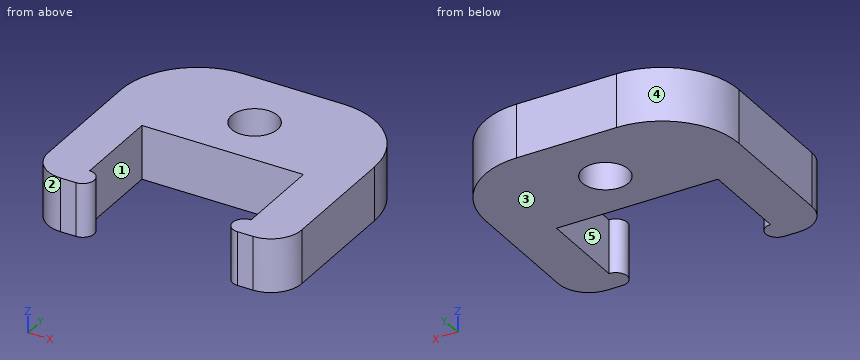
from build123d import *

# Parameters (mm, degrees)
SKETCH1_R           = 1.5
BOSS_EXTRUDE1_DEPTH = 3.5
FILLET1_R           = 2
FILLET2_R           = 5


with BuildPart() as part:
    # Sketch1 → Boss-Extrude1 (new body)
    with BuildSketch(Plane.XY):
        with BuildLine():
            Line((0, 15), (16.5, 15))
            Line((16.5, 15), (16.5, 0))
            Line((16.5, 0), (13.5, 0))
            ThreePointArc((13.5, 0), (12.75, 0.75), (13.5, 1.5))
            Line((13.5, 1.5), (13.5, 7.25))
            Line((13.5, 7.25), (3, 7.25))
            Line((3, 7.25), (3, 1.5))
            ThreePointArc((3, 1.5), (3.75, 0.75), (3, 0))
            Line((3, 0), (0, 0))
            Line((0, 0), (0, 15))
        make_face()
        with Locations((8.25, 10.75)):
            Circle(SKETCH1_R, mode=Mode.SUBTRACT)
    extrude(amount=BOSS_EXTRUDE1_DEPTH)

    # Fillet1
    fillet1_edges = [part.edges().sort_by_distance(p)[0] for p in [
        (16.5, 0, 1.75),
        (0, 0, 1.75),
    ]]
    fillet(fillet1_edges, radius=FILLET1_R)

    # Fillet2
    fillet2_edges = [part.edges().sort_by_distance(p)[0] for p in [
        (0, 15, 1.75),
        (16.5, 15, 1.75),
    ]]
    fillet(fillet2_edges, radius=FILLET2_R)


solid = part.part
Can you work these out from the model? Positions are in its coordinate system, mm. Face numbers are marked on the shaded views. A direction names the side the tool comes from. Give positions to 0.01 mm unless a question says otherwise; leave off trailing zeros. Loops run counter-clockwise (first coordinate to the right, second up) from the corner with the lowest first, then second, coordinate; pieces in that order, holes last. Notation, with made-up numbers: (17, 8.25) -> (50, 8.25) arc R16 cw to (50, 20.25) -> close; hole circle Ø1 at (32.5, 86.5). An arc over 180 degrees is marked (long way). Return JSON: item names as keys, results as strings.
Q1. For pin 1 Ø2.5 at (x, y) = (8.25, 10.75) entering from +Z, with a flat end and sliding along its axis, tell me the tip position at first contact or that it passes through.
Checks:
{"pin 1": "passes through"}
Q2. I want a section at A-A, the plane y = 4. List the corners of the cut face in (x, z) for me.
Checks:
{"outline": "(0, 0) -> (3, 0) -> (3, 3.5) -> (0, 3.5) -> close; (13.5, 0) -> (16.5, 0) -> (16.5, 3.5) -> (13.5, 3.5) -> close"}
Q3. I want a section at B-B, the plane z = 2.35. List the corners of the cut face in (x, y) for me, then the cut area to 3 significant figures.
Checks:
{"outline": "(0, 2) arc R2 ccw to (2, 0) -> (3, 0) arc R0.75 ccw to (3, 1.5) -> (3, 7.25) -> (13.5, 7.25) -> (13.5, 1.5) arc R0.75 ccw to (13.5, 0) -> (14.5, 0) arc R2 ccw to (16.5, 2) -> (16.5, 10) arc R5 ccw to (11.5, 15) -> (5, 15) arc R5 ccw to (0, 10) -> close; hole circle Ø3 at (8.25, 10.75)", "area": "154 mm2"}
Q4. I want a section at D-D, the plane x = 15.25. List the corners of the cut face in (y, z) for me.
Checks:
{"outline": "(0.15, 0) -> (13.31, 0) -> (13.31, 3.5) -> (0.15, 3.5) -> close"}
Q5. We'd pull the mould along Y, two halves only. Please class the marked faces 3, 4 and 5: released by +Y, released by -Y, zero draft, split by the parting line, or undercut.
Checks:
{"face 3": "zero draft", "face 4": "released by +Y", "face 5": "undercut"}
Q6. On a 3-axis mill with a long thin cutter (end or side, diameter ignored), from which of +Z, -Z, +X, -X, +Y, -Y can I reach the whole of each face in a straight line? I mean the marked faces 1 and 2. Say none if no direction works.
Checks:
{"face 1": "+Z, -Z", "face 2": "+Z, -Z, -X, -Y"}
Q7. I need wall thicknesses on probe 1 along X at (y, z) = (4, 1.7); probe 2 along Y at (x, z) = (8.25, 1.45); probe 3 along Y at (x, z) = (10, 1.8). Which ranges of each line are inside material? Lowest first, please.
Checks:
{"probe 1": "x = 0 to 3, 13.5 to 16.5", "probe 2": "y = 7.25 to 9.25, 12.25 to 15", "probe 3": "y = 7.25 to 15"}
Q8. I want a section at C-C, the plane x = 8.25. List the corners of the cut face in (y, z) for me, then the cut area to 3 significant figures.
Checks:
{"outline": "(7.25, 0) -> (9.25, 0) -> (9.25, 3.5) -> (7.25, 3.5) -> close; (12.25, 0) -> (15, 0) -> (15, 3.5) -> (12.25, 3.5) -> close", "area": "16.6 mm2"}
